For this review, use the dimensioned drawing (mm, ordinates from the lowest corner) and the shaded views. A direction names the side the tool comes from. Give positions to 0.01 mm unless a question says otherwise; leave off trailing zeros. Order: outer loops, then holes, each group sorted by start corner. A loop starts at its lowest first (then second) coordinate and runs counter-clockwise, first axis right, second up. Notation, with made-up numbers: M -7,-4.5 L 30,-4.5 A9 cw 30,7.5 Z; hole C 48.25,35.25 d10. An arc over 180 degrees is marked long. Use CSV: the item, a comma, the result in double quotes. Start each with the question number.
(1) Consider section A-A (x = 25.4). Write out the cut boundary in (y, z) (3 decimals).
(2) Consider section B-B (y = 8.89). Write out the cut boundary in (x, z) (3 decimals), and give its area (3 significant figures).
(3) Wall thickness on L1, parallel to X at y = 8.89, z = 36.05 (3 decimals); L2, parallel to Z at x = 3, y = 12.25 (3 decimals); L3, parallel to Y at x = 12.7, z = 37.3 (1 decimal): over which ranges is each line inside the solid? List them lowest first. Write a range as from..to.
(4) Consider section C-C (z = 19). Write out the cut boundary in (x, y).
(5) Consider section D-D (x = 44.5). Write out the cut boundary in (y, z) (3 decimals).
(6) Clearance check with flat-ended pins moving along their axes: P1, Ø15, axis at x = 25.4, z = 12.7, coming from the -Y side; P2, Ø5, axis at x = 25.5, y = 7, coming from the -Z side (3 decimals); P3, Ø10, axis at x = 38, z = 6, coming from the -Y side. State where each tip first meets the part, or that it passes through.
(7) Tool access review of the marked faces 1 and 2: name each direction out of +Z, -Z, +X, -X, +Y, -Y from which nothing blocks a thin tool from reaching the whole face with its end or side.
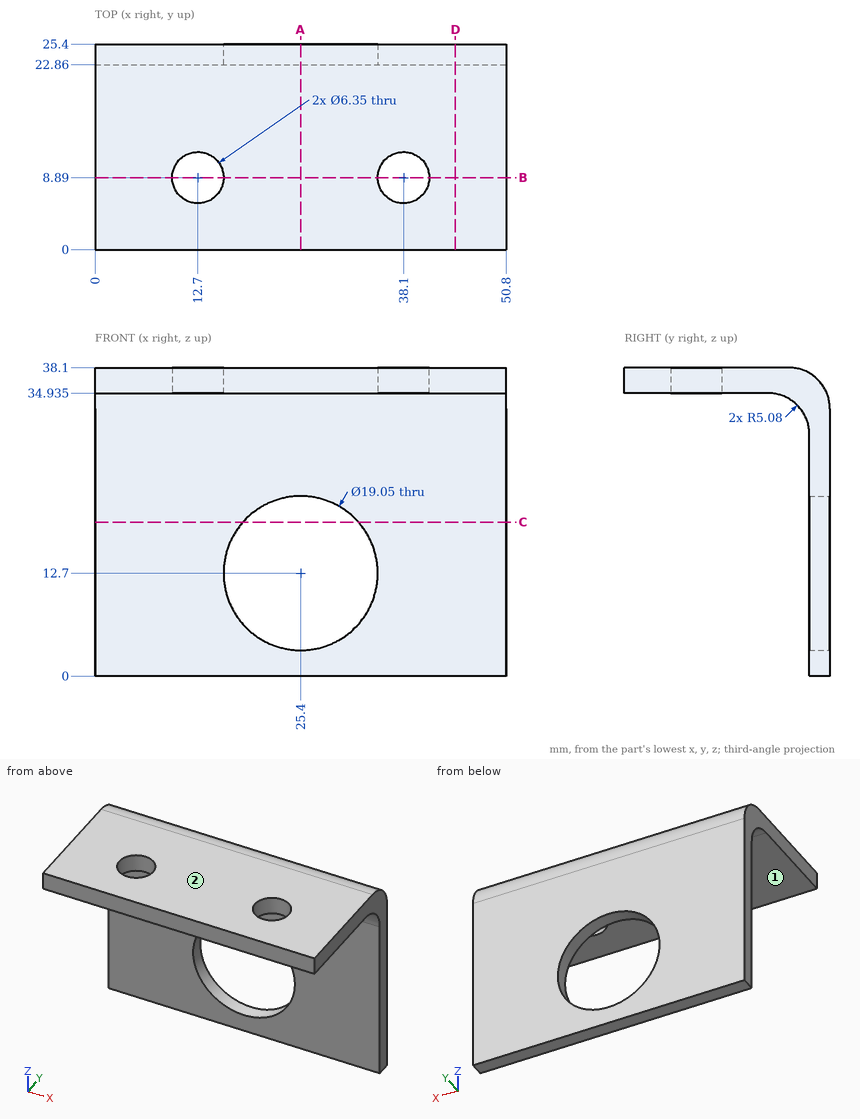
Check result:
1,outline,"M 0,34.935 L 17.78,34.935 A5.08 cw 22.86,29.855 L 22.86,22.225 L 25.4,22.225 L 25.4,33.02 A5.08 ccw 20.32,38.1 L 0,38.1 Z; M 22.86,0 L 25.4,0 L 25.4,3.175 L 22.86,3.175 Z"
2,outline,"M 0,34.935 L 9.525,34.935 L 9.525,38.1 L 0,38.1 Z; M 15.875,34.935 L 34.925,34.935 L 34.925,38.1 L 15.875,38.1 Z; M 41.275,34.935 L 50.8,34.935 L 50.8,38.1 L 41.275,38.1 Z"
2,area,"121 mm^2"
3,L1,"x = 0..9.525, 15.875..34.925, 41.275..50.8"
3,L2,"z = 34.935..38.1"
3,L3,"y = 0..5.7, 12.1..23.1"
4,outline,"M 0,22.86 L 18.26,22.86 L 18.26,25.4 L 0,25.4 Z; M 32.54,22.86 L 50.8,22.86 L 50.8,25.4 L 32.54,25.4 Z"
5,outline,"M 0,34.935 L 17.78,34.935 A5.08 cw 22.86,29.855 L 22.86,0 L 25.4,0 L 25.4,33.02 A5.08 ccw 20.32,38.1 L 0,38.1 Z"
6,P1,"passes through"
6,P2,"stops at z = 34.935"
6,P3,"stops at y = 22.86"
7,face 1,"-Z, +X, -X, -Y"
7,face 2,"+Z, +X, -X, +Y, -Y"
